Autodesk Inventor part; units mm, degrees
ref_plane "Plano de trabajo1" through (0, 0, 0) normal (0, 0, 1) x (1, 0, 0)
ref_plane "YZ Plane" through (0, 0, 0) normal (1, 0, 0) x (0, 1, 0)
ref_plane "XZ Plane" through (0, 0, 0) normal (0, 1, 0) x (-1, 0, 0)
ref_plane "Plano de trabajo1" through (0, 0, 0) normal (0, 0, 1) x (1, 0, 0)
sketch "Boceto1" plane through (0, 0, 0) normal (0, 0, 1) x (1, 0, 0)
  line L0 (-395, -200.5) -> (-395, -220.5)
  line L1 (-395, -220.5) -> (335, -220.5)
  line L2 (335, -200.5) -> (335, -220.5)
  line L3 (-395, -200.5) -> (335, -200.5)
  line L4 (-145, 767.5) -> (-145, -767.5)
  line L5 (-145, -767.5) -> (145, -767.5)
  line L6 (145, -767.5) -> (145, 767.5)
  line L7 (145, 767.5) -> (-145, 767.5)
  line L8 (335.5, -200) -> (335.5, -221)
  line L9 (335.5, -221) -> (-395.5, -221)
  line L10 (-395.5, -221) -> (-395.5, -200)
  line L11 (-395.5, -200) -> (335.5, -200)
  line L12 (-145, -200) -> (-145, -180)
  line L13 (-145, -180) -> (-125, -180)
  line L14 (-125, -180) -> (-125, -200)
  line L15 (-125, -200) -> (-145, -200)
  line L16 (-145, -200) -> (-145, -180)
  point P0 (0, 0)
  dimension "d0" = 0.5
  dimension "d1" = 20
  dimension "d2" = 20
  dimension "d3" = 20
extrude "Extrusión1" add sketch "Boceto1" along normal blind 4 contours L4 L13 L14 L11
sketch "Boceto3" plane through (0, 0, 4) normal (0, 0, 1) x (1, 0, 0)
  line L0 (-125, -180) -> (-145, -180)
  line L1 (-145, -180) -> (-145, -200)
  line L2 (-145, -200) -> (-125, -200)
  line L3 (-125, -200) -> (-125, -180)
  line L4 (-145, -200) -> (-125, -200)
  line L5 (-125, -200) -> (-125, -196)
  line L6 (-125, -196) -> (-145, -196)
  line L7 (-145, -196) -> (-145, -200)
  point P0 (0, 0)
  dimension "d6" = 4
extrude "Extrusión2" add sketch "Boceto3" along normal blind 20 contours L3 L2 L1 L6
sketch "Boceto4" plane through (-145, -200, 0) normal (0, -1, 0) x (1, 0, 0)
  line L0 (0, 0) -> (20, 0)
  line L1 (20, 0) -> (20, 24)
  line L2 (0, 24) -> (20, 24)
  line L3 (0, 0) -> (0, 24)
  line L4 (0, 24) -> (20, 24)
  line L5 (20, 24) -> (0, 24)
  line L6 (0, 24) -> (0, 20)
  line L7 (0, 20) -> (20, 20)
  line L8 (20, 20) -> (20, 24)
  point P0 (145, 0)
  dimension "d9" = 4
extrude "Extrusión3" add sketch "Boceto4" along normal blind 20.5 contours L3 L2 L1 L7
sketch "Boceto6" plane through (0, 0, 4) normal (0, 0, 1) x (1, 0, 0)
  line L0 (-145, -196) -> (-125, -196)
  line L1 (-125, -196) -> (-125, -180)
  line L2 (-125, -180) -> (-145, -180)
  line L3 (-145, -180) -> (-145, -196)
  line L4 (-145, -180) -> (-142, -180)
  line L5 (-142, -180) -> (-142, -196)
  line L6 (-142, -196) -> (-145, -196)
  line L7 (-145, -196) -> (-145, -180)
  line L8 (-125, -196) -> (-128, -196)
  line L9 (-128, -196) -> (-128, -180)
  line L10 (-128, -180) -> (-125, -180)
  line L11 (-125, -180) -> (-125, -196)
  point P0 (0, 0)
  dimension "d12" = 3
  dimension "d13" = 16
  dimension "d14" = 3
extrude "Extrusión4" add sketch "Boceto6" along normal blind 20 contours L3 L2 L5 L0 | L9 L2 L1 L0
chamfer "Chaflán1" [suppressed]
sketch "Boceto7" plane through (0, 0, 4) normal (0, 0, 1) x (1, 0, 0)
  line L0 (-142, -180) -> (-142, -196)
  line L1 (-142, -196) -> (-128, -196)
  line L2 (-128, -196) -> (-128, -180)
  line L3 (-128, -180) -> (-142, -180)
  line L4 (-138.3, -192.3) -> (-138.3, -183.7)
  line L5 (-138.3, -183.7) -> (-131.7, -183.7)
  line L6 (-131.7, -183.7) -> (-131.7, -192.3)
  line L7 (-131.7, -192.3) -> (-138.3, -192.3)
  circle A0 centre (-138.3, -183.7) radius 3
  circle A1 centre (-131.7, -192.3) radius 3
  circle A2 centre (-138.3, -183.7) radius 1.65
  circle A3 centre (-131.7, -192.3) radius 1.65
  point P0 (0, 0)
  dimension "d20" = 3.7
  dimension "d21" = 6
  dimension "d22" = 6
  dimension "d23" = 3.3
  dimension "d24" = 3.3
hole "Agujero1" at (-138.3, -183.7, 4) at (-131.7, -192.3, 4) direction (0, 0, -1) diameter 3.2 end through all countersink diameter 6 countersink angle 90
sketch "Boceto8" plane through (-145, -220.5, 0) normal (0, -1, 0) x (1, 0, 0)
  line L0 (17, 24) -> (17, 4)
  line L1 (20, 20) -> (0, 20)
  line L2 (0, 0) -> (0, 20)
  line L3 (0, 0) -> (20, 0)
  line L4 (20, 0) -> (20, 20)
  line L5 (20, 20) -> (20, 24)
  line L6 (20, 24) -> (0, 24)
  line L7 (0, 24) -> (0, 20)
  line L8 (0, 20) -> (20, 20)
  point P0 (145, 0)
extrude "Extrusión5" add sketch "Boceto8" along normal blind 3
sketch "Boceto9" plane through (0, 0, 24) normal (0, 0, 1) x (1, 0, 0)
  line L0 (-145, -180) -> (-145, -223.5)
  line L1 (-125, -223.5) -> (-145, -223.5)
  line L2 (-125, -180) -> (-125, -223.5)
  line L3 (-128, -196) -> (-142, -196)
  line L4 (-145, -223.5) -> (-125, -223.5)
  line L5 (-125, -223.5) -> (-125, -219.5)
  line L6 (-125, -219.5) -> (-145, -219.5)
  line L7 (-145, -219.5) -> (-145, -223.5)
  line L8 (-125, -180) -> (-128, -180)
  line L9 (-128, -180) -> (-128, -196)
  line L10 (-142, -196) -> (-142, -180)
  line L11 (-142, -180) -> (-145, -180)
  point P0 (0, 0)
  dimension "d35" = 4
extrude "Extrusión6" add sketch "Boceto9" along normal blind 16 contours L6 L2 L1 L0
sketch "Boceto10" plane through (-145, -219.5, 24) normal (0, 1, 0) x (1, 0, 0)
  line L0 (0, 0) -> (20, 0)
  line L1 (0, 0) -> (0, -16)
  line L2 (20, -16) -> (0, -16)
  line L3 (20, 0) -> (20, -16)
  line L4 (20, -16) -> (17, -16)
  line L5 (17, -16) -> (17, 0)
  line L6 (17, 0) -> (20, 0)
  line L7 (20, 0) -> (20, -16)
  line L8 (0, -16) -> (3, -16)
  line L9 (3, -16) -> (3, 0)
  line L10 (3, 0) -> (0, 0)
  line L11 (0, 0) -> (0, -16)
  point P0 (145, 24)
  point P1 (3, -16)
  point P2 (3, 0)
  point P3 (17, -16)
  dimension "d38" = 3
  dimension "d39" = 3
  dimension "d40" = 16
extrude "Extrusión7" add sketch "Boceto10" along normal up to surface (39.5 mm away) contours L0 L9 L2 L1 | L0 L3 L2 L5
chamfer "Chaflán2" [suppressed]
chamfer "Chaflán3" [suppressed]
sketch "Boceto11" plane through (-142, -219.5, 24) normal (0, 1, 0) x (1, 0, 0)
  line L0 (0, 0) -> (0, -16)
  line L1 (14, -16) -> (0, -16)
  line L2 (14, -16) -> (14, 0)
  line L3 (0, 0) -> (14, 0)
  line L4 (3.7, -12.3) -> (3.7, -3.7)
  line L5 (3.7, -3.7) -> (10.3, -3.7)
  line L6 (10.3, -3.7) -> (10.3, -12.3)
  line L7 (10.3, -12.3) -> (3.7, -12.3)
  circle A0 centre (3.7, -3.7) radius 1.6
  circle A1 centre (10.3, -12.3) radius 1.6
  point P0 (142, 24)
  dimension "d49" = 3.7
  dimension "d50" = 3.2
  dimension "d51" = 3.2
hole "Agujero2" at (-131.7, -219.5, 36.3) at (-138.3, -219.5, 27.7) direction (0, -1, 0) diameter 3.2 end through all countersink diameter 6 countersink angle 90
fillet "Empalme2" radius 0.5 9 edges at (-135, -219.5, 40) (-142, -207.75, 24) (-128, -207.75, 24) (-135, -219.5, 24) (-142, -196, 14) (-135, -196, 4) (-142, -188, 4) (-128, -188, 4) (-128, -196, 14)
chamfer "Chaflán4" distance 32 angle 45 2 edges at (-143.5, -180, 40) (-126.5, -180, 40)
properties part number "Uniont"
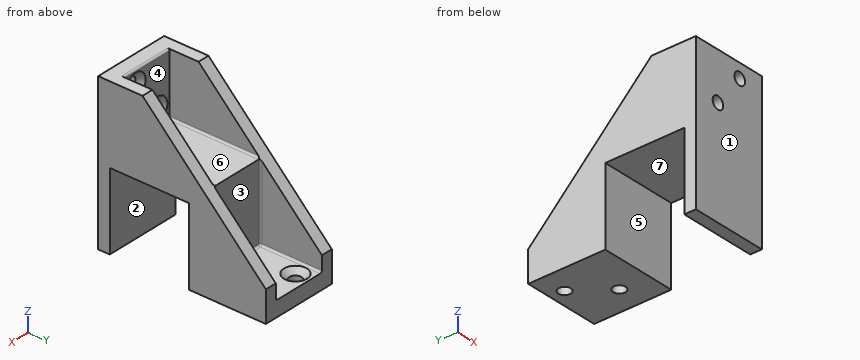
Model file for the job. Use its own axes, mm. Face numbers are marked on the shaded views. A direction names the side the tool comes from. Give positions to 0.01 mm unless a question says otherwise; leave off trailing zeros. Order: outer loops, then holes, each group sorted by start corner. A loop starts at its lowest first (then second) coordinate and runs counter-clockwise, first axis right, second up. Notation, with made-up numbers: M -24,75.5 L 26,75.5 A30 cw 26,104.5 Z; hole C -36,-5 d8. An arc over 180 degrees is marked long. Put each result on its own line as item: value. Start each with the question number.
(1) Tool access for the marked faces 1, 2 and 3: list every direction of +Z, -Z, +X, -X, +Y, -Y with a clear straight run to the whole face (end or side of a thin tool).
(2) Band-saw the part on D-D on y = -214. Give the cut face in (x, z), then the cut area to 3 significant figures.
(3) Pull direction Y, two halves, no side cores. Call the marked faces 4, 5, 6 and 7: released by +Y, released by -Y, zero draft, split by the parting line, or undercut.
(4) Pin check, flat tips, straight feed: pin 1 Ø4 at (x, z) = (-132, 35.5) entering from +Y; pin 2 Ø2.5 at (x, z) = (-131.7, 36.3) entering from +Y; pin 3 Ø8 at (y, z) = (-205, 33.5) entering from +X; pin 4 Ø4 at (x, y) = (-131.5, -201.5) entering from +Z. Stop position of each tip, or through.
(5) Drill centre lines: L1, parallel to X at y = -222, z = 27.7; L2, parallel to Y at x = -131.7, z = 1.9; L3, parallel to Z at x = -131.7, y = -221.5. Where is each one in solid material? Low to high. Write a range as [from, to].
(6) Band-saw the part on B-B on x = -131.7. Give the cut face in (y, z), then the cut area to 3 significant figures.
(7) Band-saw the part on C-C on z = 16.5. Give the cut face in (x, y), then the cut area to 3 significant figures.
(8) Band-saw the part on A-A on y = -192.3. Give the cut face in (x, z).
Results below:
1. face 1: +Z, -Z, +X, -X, -Y
1. face 2: -Z, +X, -X
1. face 3: +Z, +Y
2. outline: M -145,20 L -125,20 L -125,40 L -128,40 L -128,24.5 A0.5 cw -128.5,24 L -141.5,24 A0.5 cw -142,24.5 L -142,40 L -145,40 Z
2. area: 176 mm2
3. face 4: released by +Y
3. face 5: undercut
3. face 6: zero draft
3. face 7: undercut
4. pin 1: stops at y = -219.65
4. pin 2: passes through
4. pin 3: stops at x = -125
4. pin 4: stops at z = 24
5. L1: x = [-145, -139.9], [-136.7, -125]
5. L2: y = [-223.5, -220.5], [-200, -193.9], [-190.7, -180]
5. L3: z = [0, 34.7], [37.9, 40]
6. outline: M -223.5,0 L -220.5,0 L -220.5,20 L -200,20 L -200,0 L -193.9,0 L -193.9,2.6 L -195.3,4 L -195.5,4 A0.5 cw -196,4.5 L -196,24 L -219,24 A0.5 cw -219.5,24.5 L -219.5,33.3 L -220.9,34.7 L -223.5,34.7 Z; M -223.5,37.9 L -220.9,37.9 L -219.5,39.3 L -219.5,39.5 A0.5 ccw -220,40 L -223.5,40 Z; M -190.7,0 L -180,0 L -180,4 L -189.3,4 L -190.7,2.6 Z
6. area: 349 mm2
7. outline: M -145,-223.5 L -125,-223.5 L -125,-220.5 L -145,-220.5 Z; M -145,-200 L -125,-200 L -125,-188.5 L -128,-188.5 L -128,-195.5 A0.5 cw -128.5,-196 L -141.5,-196 A0.5 cw -142,-195.5 L -142,-188.5 L -145,-188.5 Z
7. area: 185 mm2
8. outline: M -145,0 L -133.3,0 L -133.3,2.6 L -134.7,4 L -141.5,4 A0.5 cw -142,4.5 L -142,20.3 L -145,20.3 Z; M -130.1,0 L -125,0 L -125,20.3 L -128,20.3 L -128,4.5 A0.5 cw -128.5,4 L -128.7,4 L -130.1,2.6 Z
